Geometry: final body of the model. Coordinates: model frame, mm. A direction names the side the tool comes from. Round coordinates to 2 decimals unless told otherwise and drop trailing zeros. Write each loop counter-clockwise with the first axis right and the second up, starting at its lowest first coordinate (ties: lowest second). Pieces come first, ordered by that corner, then holes. Notation, with made-up numbers: (25.25, -2.5) - (70.25, -2.5) arc R21 ccw to (70.25, 1.5) - close; hole circle Ø6 at (4.25, 72.5). An arc over 180 degrees is marked (long way). Use a Markdown table: item, result. Add a question column.
Autodesk Inventor part; units mm, degrees
ref_plane "YZ Plane" through (0, 0, 0) normal (1, 0, 0) x (0, 1, 0)
ref_plane "XZ Plane" through (0, 0, 0) normal (0, 1, 0) x (-1, 0, 0)
ref_plane "XY Plane" through (0, 0, 0) normal (0, 0, 1) x (1, 0, 0)
sketch "Sketch2" plane through (0, 0, 0) normal (0, 1, 0) x (-1, 0, 0)
  line L0 (-289.433, 50.8) -> (289.433, 50.8)
  line L1 (289.433, 50.8) -> (289.433, -50.8)
  line L2 (289.433, -50.8) -> (-289.433, -50.8)
  line L3 (-289.433, -50.8) -> (-289.433, 50.8)
  point P0 (0, 0)
  dimension "d0" = 289.433
  dimension "d1" = 289.433
  dimension "d2" = 50.8
  dimension "d3" = 50.8
extrude "Plate1" add sketch "Sketch2" along normal blind 3.048
sketch "Sketch3" plane through (-289.433, 0, 50.8) normal (0, 0, 1) x (1, 0, 0)
  arc A0 (578.866, 0) -> (585.089, 6.223) centre (578.866, 6.223) ccw
  line L0 (578.866, 6.223) -> (585.089, 6.223) construction
  line L1 (578.866, 6.223) -> (578.866, 0) construction
  line L2 (585.089, 6.223) -> (585.089, 19.5834)
  point P0 (578.866, 3.048)
  point P1 (289.433, 0)
  dimension "d5" = 90
  dimension "d6" = 6.223
  dimension "d7" = 6.223
  dimension "d8" = 13.3604
contour flange "Contour Flange1" sketch "Sketch3" thickness 3.048 bend radius 3.048 curves A0 L2 edges at (289.433, 0, 0) running between points at (289.433, 0, -50.8) (289.433, 0, 50.8)
bend "Bend1"
corner "Corner1"
sketch "Sketch4" plane through (-289.433, 0, 50.8) normal (0, 0, 1) x (1, 0, 0)
  arc A0 (-6.223, 6.223) -> (0, 0) centre (0, 6.223) ccw
  line L0 (0, 6.223) -> (-6.223, 6.223) construction
  line L1 (0, 6.223) -> (0, 0) construction
  line L2 (-6.223, 6.223) -> (-6.223, 19.5834)
  point P0 (0, 3.048)
  point P1 (289.433, 0)
  dimension "d18" = 90
  dimension "d19" = 6.223
  dimension "d20" = 6.223
  dimension "d21" = 13.3604
contour flange "Contour Flange2" sketch "Sketch4" thickness 3.048 bend radius 3.048 curves A0 L2 edges at (-289.433, 0, 0) running between points at (-289.433, 0, 50.8) (-289.433, 0, -50.8)
bend "Bend2"
corner "Corner2"
sketch "Sketch5" plane through (295.656, 6.223, -50.8) normal (1, 0, 0) x (0, 0, -1)
  line L0 (-101.6, 0) -> (-101.6, 13.3604)
  line L1 (0, -6.223) -> (-101.6, -6.223)
  point P0 (-50.8, -6.223)
  point P1 (-88.9, 6.477)
  dimension "d31" = 12.7
  dimension "d32" = 12.7
hole "Hole1" at (295.656, 12.7, 38.1) direction (-1, 0, 0) diameter 3.175 end through all
sketch "Sketch6" plane through (295.656, 6.223, -50.8) normal (1, 0, 0) x (0, 0, -1)
  circle A0 centre (-88.9, 6.477) radius 1.5875
  line L0 (-101.6, 0) -> (-101.6, 13.3604)
  line L1 (-88.9, 6.477) -> (-74.5256, 6.477)
  point P0 (-50.8, -6.223)
pattern_linear "Rectangular Pattern1" count 7 spacing 12.7 along (0, 0, -1) of "Hole1"
equation "\"d38\" = Thickness"
equation "\"d9\" = BendReliefWidth"
equation "\"d10\" = BendReliefDepth"
equation "\"d11\" = MinimumRemnant"
equation "\"d12\" = BendRadius"
equation "\"d13\" = BendRadius"
equation "\"d15\" = CornerReliefSize"
equation "\"d16\" = GapSize"
equation "\"d17\" = JacobiRadiusSize"
equation "\"d22\" = BendReliefWidth"
equation "\"d23\" = BendReliefDepth"
equation "\"d24\" = MinimumRemnant"
equation "\"d25\" = BendRadius"
equation "\"d26\" = BendRadius"
equation "\"d28\" = CornerReliefSize"
equation "\"d29\" = GapSize"
equation "\"d30\" = JacobiRadiusSize"
equation "\"BendRadius\" = Thickness"
equation "\"BendReliefWidth\" = Thickness"
equation "\"BendReliefDepth\" = 0.5 * Thickness"
equation "\"CornerReliefSize\" = 4 * Thickness"
equation "\"MinimumRemnant\" = 2 * Thickness"
equation "\"TransitionRadius\" = BendRadius"
equation "\"JacobiRadiusSize\" = BendRadius"
equation "\"GapSize\" = Thickness"
equation "\"d4\" = BendRadius"
properties part number "Base Crossbar"
1) Draft query along X for faces 3 (the flat face through (4, 3.048, -1)), 4 (the flat face through (-295.656, 14.3, -0.7)), 5 (the flat face through (295.656, 14.3, -0.7)). Return one class per face: released by +X, released by -X, zero draft, split by the parting line, or undercut.
2) Pin query (flat end, axial travel): P1, Ø3, axis at y = 12.7, z = -25.4, coming from the -X side; P2, Ø10, axis at x = -47, z = 39.5, coming from the +Y side. Return the tip coordinate at first contact, or that it passes through.
3) Material intervals for L1, parallel to X at y = 10, z = 40.5; L2, parallel to Y at x = 107, z = 38; L3, parallel to Y at x = -293.5, z = -12.7, sorted ascending. Write a range as from..to.
4) Section A-A, the plane x = -227. Return the cut outline in (y, z), then the cut area to 3 significant figures.
5) Set-up query: faces 1 (the flat face through (-292.608, 14.3, -0.7)), 2 (the flat face through (4, 0, -1)). Return all of +Z, -Z, +X, -X, +Y, -Y with unobstructed straight access to the full face (end or side cutting, diameter ignored); none if empty.
Output values:
| question | item | result |
|---|---|---|
| 1 | face 3 | undercut |
| 1 | face 4 | released by -X |
| 1 | face 5 | released by +X |
| 2 | P1 | passes through |
| 2 | P2 | stops at y = 3.05 |
| 3 | L1 | x = -295.66..-292.61, 292.61..295.66 |
| 3 | L2 | y = 0..3.05 |
| 3 | L3 | y = 1.51..11.11, 14.29..19.58 |
| 4 | outline | (0, -50.8) - (3.05, -50.8) - (3.05, 50.8) - (0, 50.8) - close |
| 4 | area | 310 mm^2 |
| 5 | face 1 | +Z, -Z, +Y |
| 5 | face 2 | +Z, -Z, +X, -X, -Y |
